```python
from build123d import *

# Parameters (mm, degrees)
SKETCH1_W           = 60
SKETCH1_H           = 4
SKETCH4_W           = 20
SKETCH4_H           = 20
BOSS_EXTRUDE2_DEPTH = 20


with BuildPart() as part:
    # Sketch1 → Revolve1 (revolve)
    with BuildSketch(Plane(origin=(0, 0, 0), x_dir=(0, 0, -1), z_dir=(1, 0, 0)), mode=Mode.PRIVATE) as revolve1_sk:
        with Locations((-15.215395953, 3.196078431)):
            Rectangle(SKETCH1_W, SKETCH1_H)
    revolve(revolve1_sk.sketch.rotate(Axis((0, 1.196078431, 45.215395953), (0, 0, -1)), 90), axis=Axis((0, 1.196078431, 45.215395953), (0, 0, -1)))

    # Sketch4 → Boss-Extrude2 (add)
    with BuildSketch(Plane.XY.offset(45.215395953)):
        with Locations((0, 1.196078431)):
            Rectangle(SKETCH4_W, SKETCH4_H)
    extrude(amount=BOSS_EXTRUDE2_DEPTH)


solid = part.part
```
Can you work these out from the model? Positions are in its coordinate system, mm. A direction names the side the tool comes from. Coordinates: 2 decimals unless noted, no trailing zeros. Loops run counter-clockwise (first coordinate to the right, second up) from the corner with the lowest first, then second, coordinate; pieces in that order, holes last. Notation, with made-up numbers: M -19,47.25 L 17,47.25 A32 cw 17,76.25 Z; hole C 72.25,65 d2. An arc over 180 degrees is marked long. Put each result on its own line as item: value. Start each with the question number.
(1) Imagine slicing it at C-C on z = 36. List the corners of the cut face in (x, y) for me.
(2) Which directions (+Z, -Z, +X, -X, +Y, -Y) give clear straight access to the entire face, cutting with the end or side of a thin tool? Please do faces 1 (the face through (-0.87, 5.1, 14.8)), 2 (the face through (-10, 1, 55)).
(3) I need wall thicknesses on probe 1 along Z at (x, y) = (-6, 1.75); probe 2 along X at (y, z) = (0.25, 8.5); probe 3 along X at (y, z) = (4.75, 35.5). Which ranges of each line are inside material? Lowest first, please.
(4) Imagine slicing it at D-D on y = -5.75. List the corners of the cut face in (x, z) for me.
(5) Imagine slicing it at A-A on x = 0. List the corners of the cut face in (y, z) for me, and give its area (3 significant figures).
(6) Will these pins go through, and if not, where does the flat tip stop? pin 1 Ø1 at (x, y) = (1, -5) entering from -Z; pin 2 Ø3 at (y, z) = (6, -1.5) entering from +X.
(7) Imagine slicing it at B-B on y = 2.5. List the corners of the cut face in (x, z) for me.
Worked answers:
1. outline: C 0,1.2 d8
2. face 1: -Z
2. face 2: +Z, -Z, -X, +Y, -Y
3. probe 1: z = 45.22 to 65.22
3. probe 2: x = -3.89 to 3.89
3. probe 3: x = -1.84 to 1.84
4. outline: M -10,45.22 L 10,45.22 L 10,65.22 L -10,65.22 Z
5. outline: M -8.8,45.22 L -2.8,45.22 L -2.8,-14.78 L 5.2,-14.78 L 5.2,45.22 L 11.2,45.22 L 11.2,65.22 L -8.8,65.22 Z
5. area: 880 mm2
6. pin 1: stops at z = 45.22
6. pin 2: stops at x = 2.25
7. outline: M -10,45.22 L -3.78,45.22 L -3.78,-14.78 L 3.78,-14.78 L 3.78,45.22 L 10,45.22 L 10,65.22 L -10,65.22 Z
